Check sheet for the drawn part. Datum: minimum x, y, z corner. Units: mm. A direction names the side the tool comes from. Round coordinates to 2 decimals unless told otherwise and drop trailing zeros. Loops run counter-clockwise (first coordinate to the right, second up) from the corner with the lowest first, then second, coordinate; pieces in that order, holes last. Notation, with made-up numbers: (-27, 67) - (8, 67) arc R17 ccw to (8, 74) - close; hole circle Ø9 at (12.25, 59.5). An arc over 180 degrees is marked (long way). Use CSV: the item, a comma, the result in double quotes.
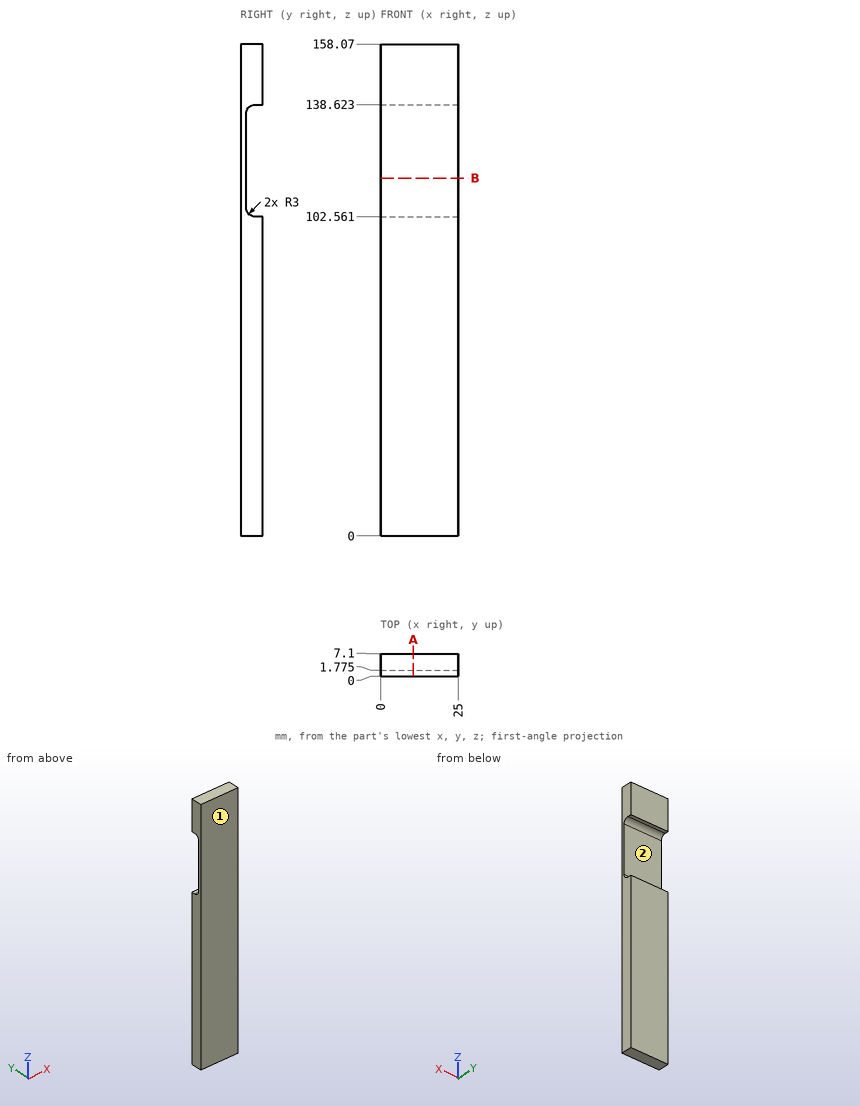
1) Thickness scan on probe 1 along Z at (x, y) = (13.25, 5.25); probe 2 along Y at (x, z) = (2, 124.5) (1 decimal); probe 3 along Z at (x, y) = (12, 3). Record the ranges inside material, lowest first. Write a range as [from, to].
Returned:
probe 1,"z = [0, 102.56], [138.62, 158.07]"
probe 2,"y = [0, 1.8]"
probe 3,"z = [0, 103.14], [138.04, 158.07]"
2) Gauge pin test, flat ends, axial feed: pin 1 Ø4 at (x, z) = (12, 106) entering from +Y; pin 2 Ø2 at (y, z) = (4, 122) entering from -X (3 decimals); pin 3 Ø12.5 at (x, z) = (8.5, 117.5) entering from +Y (3 decimals). Record the tip position at first contact, or that the pin passes through.
Returned:
pin 1,"stops at y = 2.21"
pin 2,"passes through"
pin 3,"stops at y = 1.775"
3) Cross-section at B-B, the plane z = 115. Record the cut outline in (x, y) (1 decimal).
Returned:
outline,"(0, 0) - (25, 0) - (25, 1.8) - (0, 1.8) - close"
4) Access from +Z, -Z, +X, -X, +Y, -Y to the whole of each face (thin tool, end or side, straight path). Record for the marked faces 1 and 2.
Returned:
face 1,"+Z, -Z, +X, -X, -Y"
face 2,"+X, -X, +Y"
5) Cross-section at A-A, the plane x = 10.5. Record the cut outline in (y, z) (1 decimal), then the cut area to 3 significant figures.
Returned:
outline,"(0, 0) - (7.1, 0) - (7.1, 102.6) - (4.8, 102.6) arc R3 cw to (1.8, 105.6) - (1.8, 135.6) arc R3 cw to (4.8, 138.6) - (7.1, 138.6) - (7.1, 158.1) - (0, 158.1) - close"
area,"934 mm²"
